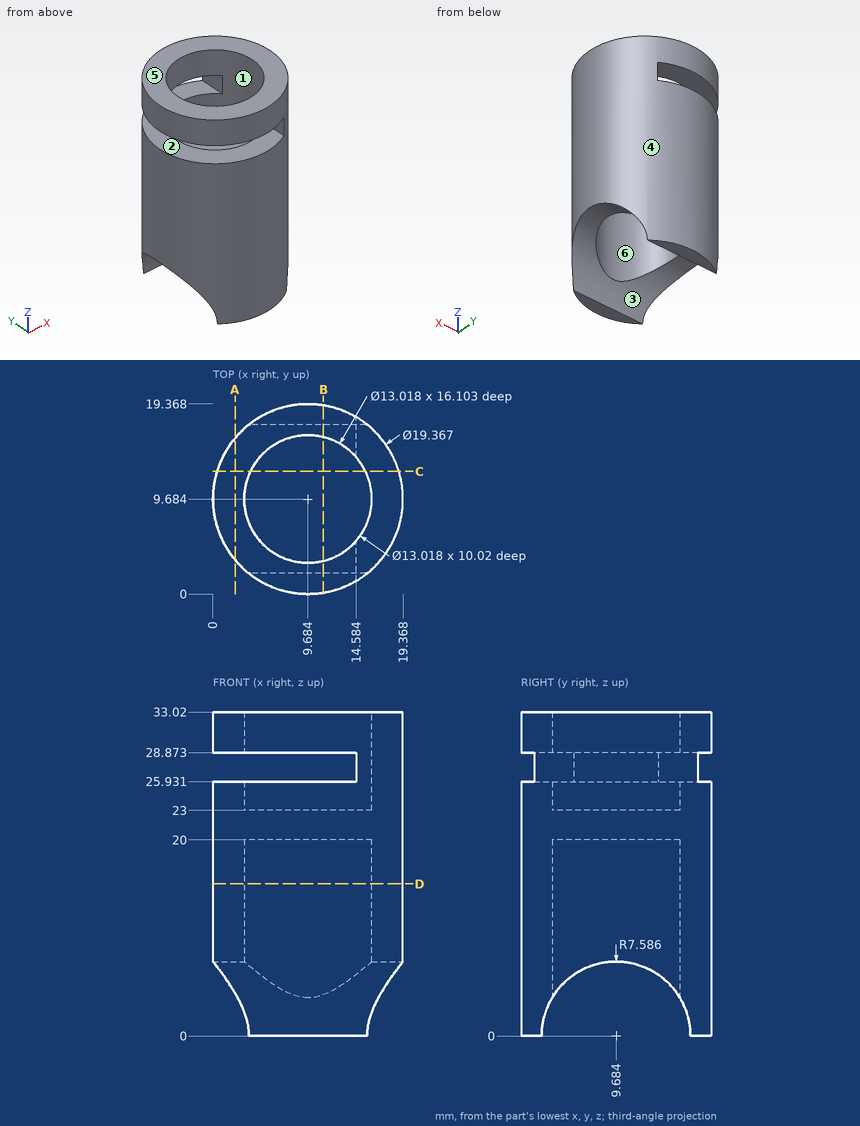
The drawing under review shows one solid part. Ordinate dimensions are in mm from its lowest x, y, z. A direction names the side the tool comes from. Round coordinates to 2 decimals unless told otherwise and drop trailing zeros. Write each loop counter-clockwise with the first axis right and the second up, starting at its lowest first coordinate (ties: lowest second). Pieces come first, ordered by that corner, then holes.
(1) Machinability: for the marked faces 1, 2 and 3, which of the approach directions +Z, -Z, +X, -X, +Y, -Y give a long, thin tool a straight path to every point of the face, cutting with its end or side? Answer none if there is none.
(2) Wall thickness on L1, parallel to X at y = 9.75, z = 31.5 (1 decimal); L2, parallel to Z at x = 4, y = 2; L3, parallel to Z at x = 6.5, y = 6.5: over which ranges is each line inside the solid? List them lowest first.
(3) Mouldability with a two-part tool opening along Y and no side actions: class the marked faces 4, 5 and 6 as +Y half, -Y half, draft (parallel to the pull), parting line (faces both ways), or undercut.
(4) We need section D-D on z = 15.5. Give the boundary of the cut face in (x, y).
(5) Insertion check: pin 1 (1.5 mm diameter, centred on y = 4.5, z = 27.5, fed in from -X); pin 2 (5 mm diameter, centred on x = 12, z = 25.5, fed in from -Y); pin 3 (4 mm diameter, centred on x = 12.5, y = 6.5, fed in from +Z); pin 4 (6 mm diameter, centred on y = 5, z = 23.5, fed in from +X). Each pin has a flat end and moves straight along its axis. Give the tip position at first contact, or say it passes through.
(6) We need section C-C on y = 12.5. Give the boundary of the cut face in (x, z) (1 decimal), and give its area (3 significant figures).
(7) We need section B-B on x = 11.25. Give the boundary of the cut face in (y, z) (1 decimal).
(8) We need section A-A on x = 2.25. Give the boundary of the cut face in (y, z) (1 decimal).
Findings below:
1. face 1: +Z
1. face 2: -X, +Y, -Y
1. face 3: -Z, +X, -X
2. L1: x = 0 to 3.2, 16.2 to 19.4
2. L2: z = 0 to 25.93, 28.87 to 33.02
2. L3: z = 20 to 23
3. face 4: parting line
3. face 5: draft
3. face 6: undercut
4. outline: circle Ø19.37 at (9.68, 9.68); hole circle Ø13.02 at (9.68, 9.68)
5. pin 1: stops at x = 14.58
5. pin 2: stops at y = 0
5. pin 3: stops at z = 23
5. pin 4: stops at x = 19.22
6. outline: (0.4, 7) - (3.8, 7) - (3.8, 20) - (15.6, 20) - (15.6, 7) - (18.9, 7) - (18.9, 33) - (15.6, 33) - (15.6, 23) - (3.8, 23) - (3.8, 25.9) - (0.4, 25.9) - close; (0.4, 28.9) - (3.8, 28.9) - (3.8, 33) - (0.4, 33) - close
6. area: 202 mm2
7. outline: (0.1, 0) - (2.1, 0) arc R7.6 cw to (3.4, 4.2) - (3.4, 20) - (16, 20) - (16, 4.2) arc R7.6 cw to (17.3, 0) - (19.2, 0) - (19.2, 25.9) - (16, 25.9) - (16, 23) - (3.4, 23) - (3.4, 25.9) - (0.1, 25.9) - close; (0.1, 28.9) - (3.4, 28.9) - (3.4, 33) - (0.1, 33) - close; (16, 28.9) - (19.2, 28.9) - (19.2, 33) - (16, 33) - close
8. outline: (3.5, 4.4) arc R7.6 cw to (15.9, 4.4) - (15.9, 25.9) - (3.5, 25.9) - close; (3.5, 28.9) - (15.9, 28.9) - (15.9, 33) - (3.5, 33) - close
